The model under review builds one solid part; all positions refer to its coordinate system, in mm. A direction names the side the tool comes from. Round coordinates to 2 decimals unless told otherwise and drop trailing zeros. Write each loop counter-clockwise with the first axis right and the second up, starting at its lowest first coordinate (ties: lowest second). Pieces come first, ordered by that corner, then holes. Notation, with made-up numbers: (35, -16.5) - (90, -16.5) arc R28 cw to (90, 13.5) - close; hole circle Ø1 at (-2, -3.75). An arc over 180 degrees is marked (long way). Return JSON: item names as keys, results as strings.
from build123d import *

# Parameters (mm, degrees)
REVOLUTION003_ANGLE                = -180
POCKET007_DEPTH                    = 80.350833
POCKET041_DEPTH                    = 1.8
SKETCH021_W                        = 20
SKETCH021_H                        = 30
POCKET009_DEPTH                    = 10.001
SKETCH022_W                        = 0.6
SKETCH022_H                        = 2
POCKET010_DEPTH                    = 0.3
SKETCH022_POLARPATTERN001_2_W      = 0.6
SKETCH022_POLARPATTERN001_2_H      = 2
POCKET010_POLARPATTERN001_2_DEPTH  = 0.3
SKETCH022_POLARPATTERN001_3_W      = 0.6
SKETCH022_POLARPATTERN001_3_H      = 2
POCKET010_POLARPATTERN001_3_DEPTH  = 0.3
SKETCH022_POLARPATTERN001_4_W      = 0.6
SKETCH022_POLARPATTERN001_4_H      = 2
POCKET010_POLARPATTERN001_4_DEPTH  = 0.3
SKETCH022_POLARPATTERN001_5_W      = 0.6
SKETCH022_POLARPATTERN001_5_H      = 2
POCKET010_POLARPATTERN001_5_DEPTH  = 0.3
SKETCH022_POLARPATTERN001_6_W      = 0.6
SKETCH022_POLARPATTERN001_6_H      = 2
POCKET010_POLARPATTERN001_6_DEPTH  = 0.3
SKETCH022_POLARPATTERN001_7_W      = 0.6
SKETCH022_POLARPATTERN001_7_H      = 2
POCKET010_POLARPATTERN001_7_DEPTH  = 0.3
SKETCH022_POLARPATTERN001_8_W      = 0.6
SKETCH022_POLARPATTERN001_8_H      = 2
POCKET010_POLARPATTERN001_8_DEPTH  = 0.3
SKETCH022_POLARPATTERN001_9_W      = 0.6
SKETCH022_POLARPATTERN001_9_H      = 2
POCKET010_POLARPATTERN001_9_DEPTH  = 0.3
SKETCH022_POLARPATTERN001_10_W     = 0.6
SKETCH022_POLARPATTERN001_10_H     = 2
POCKET010_POLARPATTERN001_10_DEPTH = 0.3
SKETCH022_POLARPATTERN001_11_W     = 0.6
SKETCH022_POLARPATTERN001_11_H     = 2
POCKET010_POLARPATTERN001_11_DEPTH = 0.3
SKETCH022_POLARPATTERN001_12_W     = 0.6
SKETCH022_POLARPATTERN001_12_H     = 2
POCKET010_POLARPATTERN001_12_DEPTH = 0.3
SKETCH022_POLARPATTERN001_13_W     = 0.6
SKETCH022_POLARPATTERN001_13_H     = 2
POCKET010_POLARPATTERN001_13_DEPTH = 0.3
FILLET006_R                        = 1.9


with BuildPart() as part:
    # Sketch011 → Revolution003 (revolve)
    with BuildSketch(Plane.XZ):
        Polygon((0, 13), (12, 13), (12, 8.5), (17, 8.5), (17, 0), (0, 0), align=None)
    revolution003 = revolve(axis=Axis((0, 0, 0), (1, 0, 0)), revolution_arc=REVOLUTION003_ANGLE)

    # Sketch017 → Pocket007 (cut, through all)
    with BuildSketch(Plane(origin=(0, 0, 0), x_dir=(-1, 0, 0), z_dir=(0, 1, 0))):
        with BuildLine():
            Line((-7, -8.375), (0, -8.375))
            Line((0, -8.375), (0, -4.625))
            Line((-7, -4.625), (0, -4.625))
            ThreePointArc((-7, -4.625), (-7.707107, -4.917893), (-8, -5.625))
            Line((-8, -7.375), (-8, -5.625))
            ThreePointArc((-8, -7.375), (-7.707107, -8.082107), (-7, -8.375))
        make_face()
    pocket007 = extrude(amount=POCKET007_DEPTH, mode=Mode.SUBTRACT)

    # Sketch024 (on XZ_Plane009 of Origin012) → Pocket041 (cut)
    with BuildSketch(Plane.XZ):
        Polygon((8, 4.4), (0, 4.4), (0, -8.4), (8, -8.4), (12.65, -3.75), (12.65, -0.25), align=None)
    pocket041 = extrude(amount=-POCKET041_DEPTH, mode=Mode.SUBTRACT)

    # Mirrored001: Revolution003, Pocket007, Pocket041 across Sketch011 V_Axis
    add(revolution003.mirror(Plane(origin=(0, 0, 0), x_dir=(0, -1, 0), z_dir=(1, 0, 0))))
    add(pocket007.mirror(Plane(origin=(0, 0, 0), x_dir=(0, -1, 0), z_dir=(1, 0, 0))), mode=Mode.SUBTRACT)
    add(pocket041.mirror(Plane(origin=(0, 0, 0), x_dir=(0, -1, 0), z_dir=(1, 0, 0))), mode=Mode.SUBTRACT)

    # Sketch021 → Pocket009 (cut, through all)
    with BuildSketch(Plane(origin=(0, 3, 0), x_dir=(-1, 0, 0), z_dir=(0, 1, 0))):
        Rectangle(SKETCH021_W, SKETCH021_H)
    extrude(amount=POCKET009_DEPTH, mode=Mode.SUBTRACT)

    # Sketch022 → Pocket010 (cut)
    with BuildSketch(Plane.YZ.offset(17)):
        with Locations((0, 7.5)):
            Rectangle(SKETCH022_W, SKETCH022_H)
    pocket010 = extrude(amount=-POCKET010_DEPTH, mode=Mode.SUBTRACT)

    # Sketch022 PolarPattern001 2 → Pocket010 PolarPattern001 2 (cut)
    with BuildSketch(Plane(origin=(17, 0, 0), x_dir=(0, 0.965926, -0.258819), z_dir=(1, 0, 0))):
        with Locations((0, 7.5)):
            Rectangle(SKETCH022_POLARPATTERN001_2_W, SKETCH022_POLARPATTERN001_2_H)
    pocket010_polarpattern001_2 = extrude(amount=-POCKET010_POLARPATTERN001_2_DEPTH, mode=Mode.SUBTRACT)

    # Sketch022 PolarPattern001 3 → Pocket010 PolarPattern001 3 (cut)
    with BuildSketch(Plane(origin=(17, 0, 0), x_dir=(0, 0.866025, -0.5), z_dir=(1, 0, 0))):
        with Locations((0, 7.5)):
            Rectangle(SKETCH022_POLARPATTERN001_3_W, SKETCH022_POLARPATTERN001_3_H)
    pocket010_polarpattern001_3 = extrude(amount=-POCKET010_POLARPATTERN001_3_DEPTH, mode=Mode.SUBTRACT)

    # Sketch022 PolarPattern001 4 → Pocket010 PolarPattern001 4 (cut)
    with BuildSketch(Plane(origin=(17, 0, 0), x_dir=(0, 0.707107, -0.707107), z_dir=(1, 0, 0))):
        with Locations((0, 7.5)):
            Rectangle(SKETCH022_POLARPATTERN001_4_W, SKETCH022_POLARPATTERN001_4_H)
    pocket010_polarpattern001_4 = extrude(amount=-POCKET010_POLARPATTERN001_4_DEPTH, mode=Mode.SUBTRACT)

    # Sketch022 PolarPattern001 5 → Pocket010 PolarPattern001 5 (cut)
    with BuildSketch(Plane(origin=(17, 0, 0), x_dir=(0, 0.5, -0.866025), z_dir=(1, 0, 0))):
        with Locations((0, 7.5)):
            Rectangle(SKETCH022_POLARPATTERN001_5_W, SKETCH022_POLARPATTERN001_5_H)
    pocket010_polarpattern001_5 = extrude(amount=-POCKET010_POLARPATTERN001_5_DEPTH, mode=Mode.SUBTRACT)

    # Sketch022 PolarPattern001 6 → Pocket010 PolarPattern001 6 (cut)
    with BuildSketch(Plane(origin=(17, 0, 0), x_dir=(0, 0.258819, -0.965926), z_dir=(1, 0, 0))):
        with Locations((0, 7.5)):
            Rectangle(SKETCH022_POLARPATTERN001_6_W, SKETCH022_POLARPATTERN001_6_H)
    pocket010_polarpattern001_6 = extrude(amount=-POCKET010_POLARPATTERN001_6_DEPTH, mode=Mode.SUBTRACT)

    # Sketch022 PolarPattern001 7 → Pocket010 PolarPattern001 7 (cut)
    with BuildSketch(Plane(origin=(17, 0, 0), x_dir=(0, 0, -1), z_dir=(1, 0, 0))):
        with Locations((0, 7.5)):
            Rectangle(SKETCH022_POLARPATTERN001_7_W, SKETCH022_POLARPATTERN001_7_H)
    pocket010_polarpattern001_7 = extrude(amount=-POCKET010_POLARPATTERN001_7_DEPTH, mode=Mode.SUBTRACT)

    # Sketch022 PolarPattern001 8 → Pocket010 PolarPattern001 8 (cut)
    with BuildSketch(Plane(origin=(17, 0, 0), x_dir=(0, -0.258819, -0.965926), z_dir=(1, 0, 0))):
        with Locations((0, 7.5)):
            Rectangle(SKETCH022_POLARPATTERN001_8_W, SKETCH022_POLARPATTERN001_8_H)
    pocket010_polarpattern001_8 = extrude(amount=-POCKET010_POLARPATTERN001_8_DEPTH, mode=Mode.SUBTRACT)

    # Sketch022 PolarPattern001 9 → Pocket010 PolarPattern001 9 (cut)
    with BuildSketch(Plane(origin=(17, 0, 0), x_dir=(0, -0.5, -0.866025), z_dir=(1, 0, 0))):
        with Locations((0, 7.5)):
            Rectangle(SKETCH022_POLARPATTERN001_9_W, SKETCH022_POLARPATTERN001_9_H)
    pocket010_polarpattern001_9 = extrude(amount=-POCKET010_POLARPATTERN001_9_DEPTH, mode=Mode.SUBTRACT)

    # Sketch022 PolarPattern001 10 → Pocket010 PolarPattern001 10 (cut)
    with BuildSketch(Plane(origin=(17, 0, 0), x_dir=(0, -0.707107, -0.707107), z_dir=(1, 0, 0))):
        with Locations((0, 7.5)):
            Rectangle(SKETCH022_POLARPATTERN001_10_W, SKETCH022_POLARPATTERN001_10_H)
    pocket010_polarpattern001_10 = extrude(amount=-POCKET010_POLARPATTERN001_10_DEPTH, mode=Mode.SUBTRACT)

    # Sketch022 PolarPattern001 11 → Pocket010 PolarPattern001 11 (cut)
    with BuildSketch(Plane(origin=(17, 0, 0), x_dir=(0, -0.866025, -0.5), z_dir=(1, 0, 0))):
        with Locations((0, 7.5)):
            Rectangle(SKETCH022_POLARPATTERN001_11_W, SKETCH022_POLARPATTERN001_11_H)
    pocket010_polarpattern001_11 = extrude(amount=-POCKET010_POLARPATTERN001_11_DEPTH, mode=Mode.SUBTRACT)

    # Sketch022 PolarPattern001 12 → Pocket010 PolarPattern001 12 (cut)
    with BuildSketch(Plane(origin=(17, 0, 0), x_dir=(0, -0.965926, -0.258819), z_dir=(1, 0, 0))):
        with Locations((0, 7.5)):
            Rectangle(SKETCH022_POLARPATTERN001_12_W, SKETCH022_POLARPATTERN001_12_H)
    pocket010_polarpattern001_12 = extrude(amount=-POCKET010_POLARPATTERN001_12_DEPTH, mode=Mode.SUBTRACT)

    # Sketch022 PolarPattern001 13 → Pocket010 PolarPattern001 13 (cut)
    with BuildSketch(Plane(origin=(17, 0, 0), x_dir=(0, -1, 0), z_dir=(1, 0, 0))):
        with Locations((0, 7.5)):
            Rectangle(SKETCH022_POLARPATTERN001_13_W, SKETCH022_POLARPATTERN001_13_H)
    pocket010_polarpattern001_13 = extrude(amount=-POCKET010_POLARPATTERN001_13_DEPTH, mode=Mode.SUBTRACT)

    # Mirrored005: Pocket010, Pocket010 PolarPattern001 2, Pocket010 PolarPattern001 3, Pocket010 PolarPattern001 4, Pocket010 PolarPattern001 5, Pocket010 PolarPattern001 6, Pocket010 PolarPattern001 7, Pocket010 PolarPattern001 8, Pocket010 PolarPattern001 9, Pocket010 PolarPattern001 10, Pocket010 PolarPattern001 11, Pocket010 PolarPattern001 12, Pocket010 PolarPattern001 13 across YZ
    add(pocket010.mirror(Plane.YZ), mode=Mode.SUBTRACT)
    add(pocket010_polarpattern001_2.mirror(Plane.YZ), mode=Mode.SUBTRACT)
    add(pocket010_polarpattern001_3.mirror(Plane.YZ), mode=Mode.SUBTRACT)
    add(pocket010_polarpattern001_4.mirror(Plane.YZ), mode=Mode.SUBTRACT)
    add(pocket010_polarpattern001_5.mirror(Plane.YZ), mode=Mode.SUBTRACT)
    add(pocket010_polarpattern001_6.mirror(Plane.YZ), mode=Mode.SUBTRACT)
    add(pocket010_polarpattern001_7.mirror(Plane.YZ), mode=Mode.SUBTRACT)
    add(pocket010_polarpattern001_8.mirror(Plane.YZ), mode=Mode.SUBTRACT)
    add(pocket010_polarpattern001_9.mirror(Plane.YZ), mode=Mode.SUBTRACT)
    add(pocket010_polarpattern001_10.mirror(Plane.YZ), mode=Mode.SUBTRACT)
    add(pocket010_polarpattern001_11.mirror(Plane.YZ), mode=Mode.SUBTRACT)
    add(pocket010_polarpattern001_12.mirror(Plane.YZ), mode=Mode.SUBTRACT)
    add(pocket010_polarpattern001_13.mirror(Plane.YZ), mode=Mode.SUBTRACT)

    # Fillet006
    fillet006_edges = [part.edges().sort_by_distance(p)[0] for p in [
        (-10, 3, 0),
        (10, 3, 0),
    ]]
    fillet(fillet006_edges, radius=FILLET006_R)


solid = part.part
(1) Wall thickness on line 1 (X direction, y = 8, z = -5.5); line 2 (X direction, y = 6.25, z = 1); line 3 (Y direction, x = -5.5, z = -10): over which ranges is each line inside the solid? List them lowest first.
Filled in:
{"line 1": "x = -12 to -10, 10 to 12", "line 2": "x = -17 to -10, 10 to 17", "line 3": "y = 0 to 3"}
(2) Mouldability with a two-part tool opening along Y and no side actions: class faces 1 (the flat face through (17, 3, 0)), 2 (the flat face through (-16.85, 4, -6.33)), 3 (the flat face through (-16.7, 4, 7)), 4 (the flat face through (0, 1.8, 0)) as released by +Y, released by -Y, zero draft, split by the parting line, or undercut.
Filled in:
{"face 1": "zero draft", "face 2": "undercut", "face 3": "undercut", "face 4": "released by -Y"}
(3) Add section B-B (y = 11). Write out the cut boundary in (x, z).
Filled in:
{"outline": "(-12, -6.93) - (-10, -6.93) - (-10, 6.93) - (-12, 6.93) - close; (10, -6.93) - (12, -6.93) - (12, 6.93) - (10, 6.93) - close"}
(4) For faces 5 (the flat face through (-16.7, 7, 4)), 6 (the flat face through (0, 2, -8.375)), 7 (the flat face through (-17, 3, 0)), 8 (the flat face through (12.65, 1, -2)), 9 (the flat face through (16.7, 4, 7)), list the 3-axis set-ups (+Z, -Z, +X, -X, +Y, -Y) from which the entire face can be reached by the end or side of a thin tool; tool diameter is ignored.
Filled in:
{"face 5": "-X", "face 6": "+Y, -Y", "face 7": "+Z, -Z, -X, +Y, -Y", "face 8": "-Y", "face 9": "+X"}
(5) Add section D-D (z = -1). Write out the cut boundary in (x, y), plus the area to 3 significant figures.
Filled in:
{"outline": "(-17, 0) - (-12.65, 0) - (-12.65, 1.8) - (12.65, 1.8) - (12.65, 0) - (17, 0) - (17, 8.44) - (12, 8.44) - (12, 12.96) - (10, 12.96) - (10, 4.9) arc R1.9 cw to (8.1, 3) - (-8.1, 3) arc R1.9 cw to (-10, 4.9) - (-10, 12.96) - (-12, 12.96) - (-12, 8.44) - (-17, 8.44) - close", "area": "152 mm2"}
(6) Add section A-A (x = -4.5). Write out the cut boundary in (y, z) (3 decimals).
Filled in:
{"outline": "(0, -13) arc R13 ccw to (3, -12.649) - (3, -8.375) - (1.8, -8.375) - (1.8, -8.4) - (0, -8.4) - close; (0, 4.4) - (1.8, 4.4) - (1.8, -4.625) - (3, -4.625) - (3, 12.649) arc R13 ccw to (0, 13) - close"}
(7) Add section C-C (y = 1). Write out the cut boundary in (x, z).
Filled in:
{"outline": "(-17, -8.44) - (-12, -8.44) - (-12, -12.96) - (12, -12.96) - (12, -8.44) - (17, -8.44) - (17, 8.44) - (12, 8.44) - (12, 12.96) - (-12, 12.96) - (-12, 8.44) - (-17, 8.44) - close; hole (-12.65, -3.75) - (-8, -8.4) - (8, -8.4) - (12.65, -3.75) - (12.65, -0.25) - (8, 4.4) - (-8, 4.4) - (-12.65, -0.25) - close"}
(8) Clearance check with flat-ended pins moving along their axes: pin 1 Ø3 at (y, z) = (5.5, -9) entering from +X; pin 2 Ø0.5 at (y, z) = (2, -7) entering from -X; pin 3 Ø13 at (x, z) = (1.5, 1) entering from +Y; pin 4 Ø4 at (x, z) = (-12.5, 7.5) entering from +Y. State where each tip first meets the part, or that it passes through.
Filled in:
{"pin 1": "stops at x = 12", "pin 2": "stops at x = -17", "pin 3": "stops at y = 3", "pin 4": "stops at y = 11.75"}
